```python
from build123d import *

# Parameters (mm, degrees)
F0_W     = 50.8
F0_H     = 76.2
F1_DEPTH = 25.4
F2_R     = 5.08
F3_R     = 4.94494
F4_DEPTH = 25.4
F5_R     = 5.08
F6_R     = 6.503178
F6_R_2   = 6.191373
F7_DEPTH = 5.08


with BuildPart() as f1:
    # F0 (on Top) → F1 (new body)
    with BuildSketch(Plane.XY):
        with Locations((25.4, -38.1)):
            Rectangle(F0_W, F0_H)
    extrude(amount=F1_DEPTH)

    # F2
    f2_edges = [f1.edges().sort_by_distance(p)[0] for p in [
        (0, -76.2, 12.7),
        (50.8, -76.2, 12.7),
        (50.8, 0, 12.7),
        (0, 0, 12.7),
    ]]
    fillet(f2_edges, radius=F2_R)

    # F3 (on face) → F4 (cut)
    with BuildSketch(Plane.XZ.offset(76.2)):
        with Locations((15.094488, 12.532027)):
            Circle(F3_R)
    extrude(amount=-F4_DEPTH, mode=Mode.SUBTRACT)

    # F5
    f5_edges = [f1.edges().sort_by_distance(p)[0] for p in [
        (25.4, -76.2, 25.4),
        (25.4, -76.2, 0),
    ]]
    fillet(f5_edges, radius=F5_R)

    # F6 (on face) → F7 (cut)
    with BuildSketch(Plane.XY):
        with Locations((26.003035, -15.508536)):
            Circle(F6_R)
        with Locations((26.003035, -15.508536)):
            Circle(F6_R_2, mode=Mode.SUBTRACT)
    extrude(amount=F7_DEPTH, mode=Mode.SUBTRACT)


solid = f1.part
```
Model file for the job. Use its own axes, mm. A direction names the side the tool comes from. Coordinates: 2 decimals unless noted, no trailing zeros. Write each loop counter-clockwise with the first axis right and the second up, starting at its lowest first coordinate (ties: lowest second). Pieces come first, ordered by that corner, then holes. Notation, with made-up numbers: (75, 63.5) - (111, 63.5) arc R15 ccw to (111, 80.5) - close; hole circle Ø2 at (-37.5, 36.5). An arc over 180 degrees is marked (long way). Use a Markdown table: item, result. Add a question column.
Item 1: Drop a flat-ended pin along its axis: pin 1 (5 mm diameter, centred on x = 15.5, z = 12.5, fed in from -Y). Give the stop position or say it passes through.
Item 2: Band-saw the part on B-B, the plane z = 9.75. Write the cut outline in (x, y), and give its area (3 significant figures).
Item 3: Band-saw the part on D-D, the plane x = 14. Write the cut outline in (y, z), and give its area (3 significant figures).
Item 4: Band-saw the part on A-A, the plane y = -29. Write the cut outline in (x, z), and give its area (3 significant figures).
Item 5: Band-saw the part on C-C, the plane y = -54. Write the cut outline in (x, z).
Item 6: Drill centre lines: line 1 along Y through (x, z) = (29, 2); line 2 along Z through (x, y) = (18.5, -59.5); line 3 along Y through (x, z) = (35.5, 4). Where is each one in solid material? Low to high.
Item 7: 3-axis set-ups, long thin cutter, end or side, ignore diameter. For faces 1 (the face through (21.21, -11.113, 2.504)), 2 (the face through (49.272, -37.638, 1.449)): which of +Z, -Z, +X, -X, +Y, -Y reach the whole face in a straight line?
Item 8: Two-plate mould, pull along Y, no slides. Class faces 3 (the face through (15, -50.8, 13)), 4 (the face through (25.116, -1.528, 1.449)), 5 (the face through (31.722, -17.88, 2.504)): pulls with the +Y half, pulls with the -Y half, needs draft (parallel to the pull), parting line crosses it, or undercut.
A:
| question | item | result |
|---|---|---|
| 1 | pin 1 | stops at y = -50.8 |
| 2 | outline | (0, -71.12) arc R5.08 ccw to (5.08, -76.2) - (11.01, -76.2) - (11.01, -50.8) - (19.18, -50.8) - (19.18, -76.2) - (45.72, -76.2) arc R5.08 ccw to (50.8, -71.12) - (50.8, -5.08) arc R5.08 ccw to (45.72, 0) - (5.08, 0) arc R5.08 ccw to (0, -5.08) - close |
| 2 | area | 3,640 mm² |
| 3 | outline | (-76.2, 5.08) arc R5.08 ccw to (-71.12, 0) - (-5.08, 0) arc R5.08 ccw to (0, 5.08) - (0, 20.32) arc R5.08 ccw to (-5.08, 25.4) - (-71.12, 25.4) arc R5.08 ccw to (-76.2, 20.32) - (-76.2, 17.35) - (-50.8, 17.35) - (-50.8, 7.71) - (-76.2, 7.71) - close |
| 3 | area | 1,670 mm² |
| 4 | outline | (0, 5.08) arc R5.08 ccw to (5.08, 0) - (45.72, 0) arc R5.08 ccw to (50.8, 5.08) - (50.8, 20.32) arc R5.08 ccw to (45.72, 25.4) - (5.08, 25.4) arc R5.08 ccw to (0, 20.32) - close |
| 4 | area | 1,270 mm² |
| 5 | outline | (0, 5.08) arc R5.08 ccw to (5.08, 0) - (45.72, 0) arc R5.08 ccw to (50.8, 5.08) - (50.8, 20.32) arc R5.08 ccw to (45.72, 25.4) - (5.08, 25.4) arc R5.08 ccw to (0, 20.32) - close; hole circle Ø9.89 at (15.09, 12.53) |
| 6 | line 1 | y = -75.16 to -21.28, -20.93 to -10.09, -9.74 to -1.04 |
| 6 | line 2 | z = 0 to 8.95, 16.12 to 25.4 |
| 6 | line 3 | y = -76.08 to -0.12 |
| 7 | face 1 | -Z |
| 7 | face 2 | -Z, +X, +Y, -Y |
| 8 | face 3 | pulls with the -Y half |
| 8 | face 4 | pulls with the +Y half |
| 8 | face 5 | undercut |
